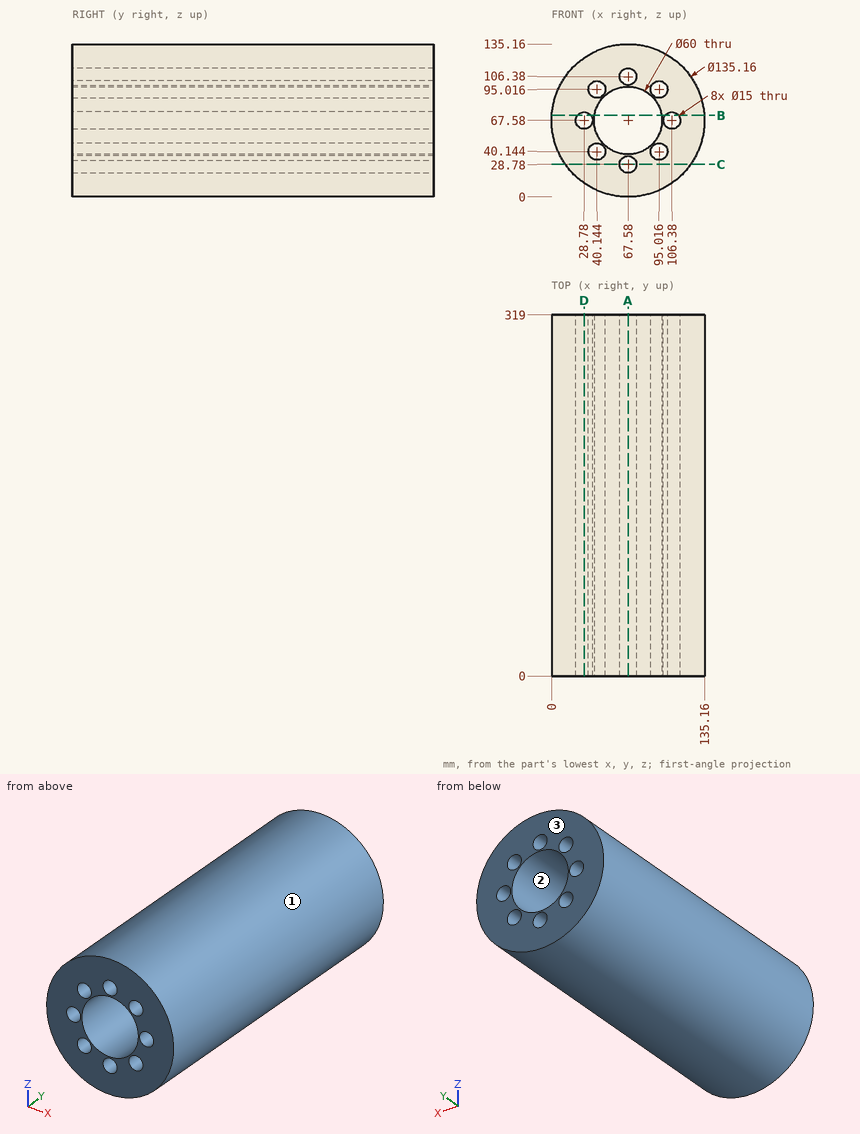
For this review, use the dimensioned drawing (mm, ordinates from the lowest corner) and the shaded views. Coordinates: 2 decimals unless noted, no trailing zeros. Order: outer loops, then holes, each group sorted by start corner. A loop starts at its lowest first (then second) coordinate and runs counter-clockwise, first axis right, second up. Notation, with made-up numbers: (42, 59) -> (47, 59) arc R16 cw to (47, 80) -> close; hole circle Ø8 at (-13, -7.75). An arc over 180 degrees is marked (long way). One line per item, written item: value. Start each with the question number.
Q1. Take a section at D-D, the plane x = 28.78. State the section outline as (y, z) points, then the cut area to 3 significant figures.
Q2. Take a section at A-A, the plane x = 67.58. State the section outline as (y, z) points.
Q3. Mouldability with a two-part tool opening along X and no side actions: class the marked faces 1, 2 and 3 as pulls with the +X half, pulls with the -X half, needs draft (parallel to the pull), parting line crosses it, or undercut.
Q4. For probe 1 along X at (y, z) = (136, 67) (1 decimal); probe 2 along Z at (x, y) = (67, 196); probe 3 along X at (y, z) = (109, 91.5) (1 decimal), list the stretches that pass through material, from the lowest coordinate up.
Q5. Insertion check: pin 1 Ø12 at (x, y) = (112, 47) entering from -Z; pin 2 Ø10 at (x, y) = (86.5, 147) entering from +Z; pin 3 Ø1.5 at (y, z) = (152, 115.5) entering from -X (1 decimal). Each pin has a flat end and moves straight along its axis. Give the tip position at first contact, or say it passes through.
Q6. Take a section at B-B, the plane z = 72. State the section outline as (x, y) points (1 decimal), then the cut area to 3 significant figures.
Q7. Take a section at C-C, the plane z = 28.78. State the section outline as (x, y) points.
Values follow:
1. outline: (0, 12.25) -> (319, 12.25) -> (319, 60.08) -> (0, 60.08) -> close; (0, 75.08) -> (319, 75.08) -> (319, 122.91) -> (0, 122.91) -> close
1. area: 30,500 mm2
2. outline: (0, 0) -> (319, 0) -> (319, 21.28) -> (0, 21.28) -> close; (0, 36.28) -> (319, 36.28) -> (319, 37.58) -> (0, 37.58) -> close; (0, 97.58) -> (319, 97.58) -> (319, 98.88) -> (0, 98.88) -> close; (0, 113.88) -> (319, 113.88) -> (319, 135.16) -> (0, 135.16) -> close
3. face 1: parting line crosses it
3. face 2: undercut
3. face 3: needs draft
4. probe 1: x = 0 to 21.3, 36.3 to 37.6, 97.6 to 98.9, 113.9 to 135.2
4. probe 2: z = 0 to 21.3, 36.26 to 37.59, 97.57 to 98.9, 113.86 to 135.16
4. probe 3: x = 4.4 to 33.5, 46.8 to 49.5, 85.7 to 88.4, 101.6 to 130.8
5. pin 1: stops at z = 11.98
5. pin 2: stops at z = 133.71
5. pin 3: stops at x = 19.2
6. outline: (0.1, 0) -> (22.7, 0) -> (22.7, 319) -> (0.1, 319) -> close; (34.8, 0) -> (37.9, 0) -> (37.9, 319) -> (34.8, 319) -> close; (97.3, 0) -> (100.3, 0) -> (100.3, 319) -> (97.3, 319) -> close; (112.4, 0) -> (135, 0) -> (135, 319) -> (112.4, 319) -> close
6. area: 16,400 mm2
7. outline: (12.25, 0) -> (60.08, 0) -> (60.08, 319) -> (12.25, 319) -> close; (75.08, 0) -> (122.91, 0) -> (122.91, 319) -> (75.08, 319) -> close
